Could you check a few things on this model? Use its own coordinates, in mm. Face numbers are marked on the shaded views. A direction names the side the tool comes from. Give positions to 0.01 mm unless a question says otherwise; leave off trailing zeros. Loops run counter-clockwise (first coordinate to the right, second up) from the corner with the lowest first, then second, coordinate; pieces in that order, holes last. Notation, with made-up numbers: M 21.25,-37.75 L 31.25,-37.75 A5 cw 31.25,-28.75 Z; hole C -13,37 d5. An arc over 180 degrees is marked long. Answer in a Markdown table with one row per item. Add a question column.
1. I need wall thicknesses on line 1 along Y through (x, z) = (0, -0.75); line 2 along X through (y, z) = (-444, -2); line 3 along Z through (x, y) = (-1, -203). Which ranges of each line are inside material? Lowest first, please. Write a range as from..to.
2. Which directions (+Z, -Z, +X, -X, +Y, -Y) give clear straight access to the entire face, cutting with the end or side of a thin tool? Please do the marked faces 1, 2, 3, 4 and 5.
3. If we section it at C-C on y = -174: List the corners of the cut face in (x, z) for me, then the cut area to 3 significant figures.
4. I'm going to push flat-ended pins straight in: pin 1 Ø17.5 at (x, z) = (4.5, 41) entering from +Y; pin 2 Ø12 at (x, z) = (38, 95) entering from +Y; pin 3 Ø6 at (x, y) = (-2.5, -286.5) entering from +Z; pin 4 Ø16.5 at (x, y) = (0, -444.5) entering from -Z. Where does each tip first touch, or does it pass through?
5. Thinking about a two-plate mould opening in Z: for the marked faces 6, 7 and 8, which applies, released by +Z, released by -Z, zero draft, split by the parting line, or undercut?
6. If we section it at B-B on y = -444.5: List the corners of the cut face in (x, z) for me, then the cut area to 3 significant figures.
7. If we section it at A-A on x = 0: List the corners of the cut face in (y, z) for me, then the cut area to 3 significant figures.
8. If we section it at D-D on z = 74.5: List the corners of the cut face in (x, y) for me.
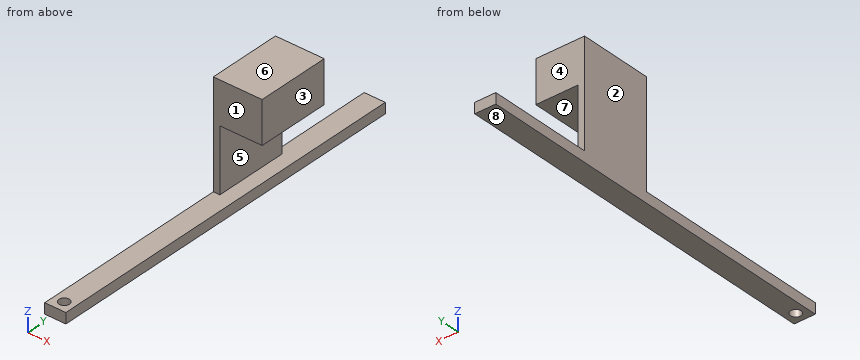
```python
from build123d import *

# Parameters (mm, degrees)
F0_W     = 25.4
F0_H     = 12.7
F1_DEPTH = 457.2
F2_W     = 7.9248
F2_H     = 88.9
F3_DEPTH = 127
F4_W     = 88.9
F4_H     = 50.8
F5_DEPTH = 50.8
F6_R     = 6.35
F7_DEPTH = 25.4


with BuildPart() as f1:
    # F0 (on Front) → F1 (new body)
    with BuildSketch(Plane.XZ):
        Rectangle(F0_W, F0_H)
    extrude(amount=F1_DEPTH)

    # F2 (on face) → F3 (join)
    with BuildSketch(Plane.XY.offset(6.35)):
        with Locations((-8.7376, -171.45)):
            Rectangle(F2_W, F2_H)
    extrude(amount=F3_DEPTH)

    # F4 (on face) → F5 (join)
    with BuildSketch(Plane.YZ.offset(-4.7752)):
        with Locations((-171.45, 107.95)):
            Rectangle(F4_W, F4_H)
    extrude(amount=F5_DEPTH)

    # F6 (on face) → F7 (cut)
    with BuildSketch(Plane.XY.offset(6.35)):
        with Locations((0, -444.5)):
            Circle(F6_R)
    extrude(amount=-F7_DEPTH, mode=Mode.SUBTRACT)


solid = f1.part
```
Results:
| question | item | result |
|---|---|---|
| 1 | line 1 | -457.2..-450.85, -438.15..0 |
| 1 | line 2 | -12.7..-6.33, 6.33..12.7 |
| 1 | line 3 | -6.35..6.35, 82.55..133.35 |
| 2 | face 1 | +Z, +X, -X, -Y |
| 2 | face 2 | +Z, -Z, -X, +Y, -Y |
| 2 | face 3 | +Z, -Z, +X, +Y, -Y |
| 2 | face 4 | +Z, +X, -X, +Y |
| 2 | face 5 | +X, +Y, -Y |
| 3 | outline | M -12.7,-6.35 L 12.7,-6.35 L 12.7,6.35 L -4.78,6.35 L -4.78,82.55 L 46.02,82.55 L 46.02,133.35 L -12.7,133.35 Z |
| 3 | area | 3,910 mm2 |
| 4 | pin 1 | through |
| 4 | pin 2 | y = -127 |
| 4 | pin 3 | z = 6.35 |
| 4 | pin 4 | z = -6.35 |
| 5 | face 6 | released by +Z |
| 5 | face 7 | undercut |
| 5 | face 8 | released by -Z |
| 6 | outline | M -12.7,-6.35 L -6.35,-6.35 L -6.35,6.35 L -12.7,6.35 Z; M 6.35,-6.35 L 12.7,-6.35 L 12.7,6.35 L 6.35,6.35 Z |
| 6 | area | 161 mm2 |
| 7 | outline | M -457.2,-6.35 L -450.85,-6.35 L -450.85,6.35 L -457.2,6.35 Z; M -438.15,-6.35 L 0,-6.35 L 0,6.35 L -438.15,6.35 Z; M -215.9,82.55 L -127,82.55 L -127,133.35 L -215.9,133.35 Z |
| 7 | area | 10,200 mm2 |
| 8 | outline | M -12.7,-215.9 L -4.78,-215.9 L -4.78,-127 L -12.7,-127 Z |
